from build123d import *

# Parameters (mm, degrees)
F0_W     = 24
F0_H     = 16
F1_DEPTH = 24


with BuildPart() as f1:
    # F0 (on Front) → F1 (new body, symmetric)
    with BuildSketch(Plane.XZ):
        Polygon((19.676238, 0), (-40.323762, 0), (-40.323762, -32), (67.676238, -32), (67.676238, 16), (67.676238, 24), (55.676238, 24), (55.676238, 32), (31.676238, 32), (31.676238, 24), (19.676238, 24), align=None)
        with Locations((43.676238, 8)):
            Rectangle(F0_W, F0_H, mode=Mode.SUBTRACT)
    extrude(amount=F1_DEPTH, both=True)


solid = f1.part
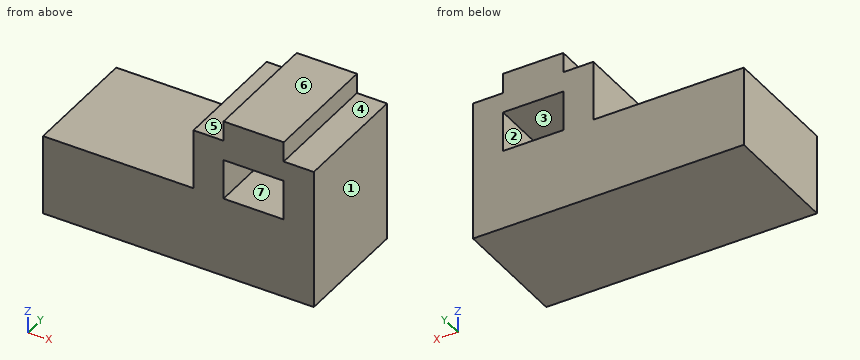
Verification items for the finished model (mm, model axes). Face numbers are marked on the shaded views. A direction names the side the tool comes from. Give positions to 0.01 mm unless a question says otherwise; leave off trailing zeros. Order: outer loops, then holes, each group sorted by start corner. A loop starts at its lowest first (then second) coordinate and runs counter-clockwise, first axis right, second up. Notation, with made-up numbers: M 44.5,29 L 64.5,29 A22 ccw 64.5,46 Z; hole C -38.5,-33.75 d11. An arc over 180 degrees is marked long. Answer as a JSON object with one key per item and string values. Group by question number.
1) Scan lines: line 1 along X through (y, z) = (-15.5, 7); line 2 along Z through (x, y) = (51, -18.5); line 3 along Z through (x, y) = (57.5, -19.5). Record each from-to range of solid material in increasing order. Write a range as [from, to].
2) Cross-section at B-B (y = 6.5). Enter the section's corners in (x, z), then the cut area to 3 significant figures.
3) Mould release check, pull along X, two halves, no side actions. Record for the marked faces 1, 2, 3 and 4: released by +X, released by -X, zero draft, split by the parting line, or undercut.
4) Access from +Z, -Z, +X, -X, +Y, -Y to the whole of each face (thin tool, end or side, straight path). Record for the marked faces 5, 6 and 7.
5) Cross-section at D-D (x = 2.5). Enter the section's corners in (y, z), then the cut area to 3 significant figures.
6) Cross-section at C-C (x = 60.5). Enter the section's corners in (y, z), then the cut area to 3 significant figures.
7) Cross-section at A-A (z = 6.5). Enter the section's corners in (x, y), then the cut area to 3 significant figures.
8) Depth check by flat-ended pin: pin 1 Ø6 at (x, y) = (27.5, -6) entering from +Z; pin 2 Ø4 at (x, z) = (12, 1.5) entering from +Y; pin 3 Ø24 at (x, y) = (-3, -6) entering from +Z; pin 4 Ø5 at (y, z) = (6.5, 21) entering from -X. Enter the tip coordinate at first touch or a pass-through.
Result sheet:
{
 "1": {"line 1": "x = [19.68, 31.68], [55.68, 67.68]", "line 2": "z = [-32, 0], [16, 32]", "line 3": "z = [-32, 24]"},
 "2": {"outline": "M -40.32,-32 L 67.68,-32 L 67.68,24 L 55.68,24 L 55.68,32 L 31.68,32 L 31.68,24 L 19.68,24 L 19.68,0 L -40.32,0 Z; hole M 31.68,0 L 55.68,0 L 55.68,16 L 31.68,16 Z", "area": "4,420 mm2"},
 "3": {"face 1": "released by +X", "face 2": "undercut", "face 3": "undercut", "face 4": "zero draft"},
 "4": {"face 5": "+Z, -X, +Y, -Y", "face 6": "+Z, +X, -X, +Y, -Y", "face 7": "+Y, -Y"},
 "5": {"outline": "M -24,-32 L 24,-32 L 24,0 L -24,0 Z", "area": "1,540 mm2"},
 "6": {"outline": "M -24,-32 L 24,-32 L 24,24 L -24,24 Z", "area": "2,690 mm2"},
 "7": {"outline": "M 19.68,-24 L 31.68,-24 L 31.68,24 L 19.68,24 Z; M 55.68,-24 L 67.68,-24 L 67.68,24 L 55.68,24 Z", "area": "1,150 mm2"},
 "8": {"pin 1": "stops at z = 24", "pin 2": "stops at y = 24", "pin 3": "stops at z = 0", "pin 4": "stops at x = 19.68"}
}
